from build123d import *

# Parameters (mm, degrees)
ESBO_O1_R                = 18
RESSALTO_EXTRUS_O1_DEPTH = 27
ESBO_O7_R                = 3.5
ESBO_O7_R_2              = 3
CORTE_EXTRUS_O3_DEPTH    = 5
ESBO_O13_R               = 3.5
ESBO_O13_R_2             = 1.25
CORTE_EXTRUS_O4_DEPTH    = 5
ESBO_O14_R               = 6.5
RESSALTO_EXTRUS_O2_DEPTH = 1.6
RESSALTO_EXTRUS_O4_DEPTH = 7
CORTE_EXTRUS_O5_DEPTH    = 7
ESBO_O21_R               = 1.25
RESSALTO_EXTRUS_O5_DEPTH = 7
CORTE_EXTRUS_O6_START    = -1
ESBO_O22_R               = 3.5
CORTE_EXTRUS_O6_DEPTH    = 1
ESBO_O23_R               = 2.5
RESSALTO_EXTRUS_O6_DEPTH = 17.5
FILETE2_R                = 0.5


with BuildPart() as part:
    # Esboço1 → Ressalto-extrusão1 (new, symmetric)
    with BuildSketch(Plane.XY):
        Circle(ESBO_O1_R)
    extrude(amount=RESSALTO_EXTRUS_O1_DEPTH, both=True)

    # Esboço7 → Corte-extrusão3 (cut)
    with BuildSketch(Plane(origin=(0, 0, -27), x_dir=(-1, 0, 0), z_dir=(0, 0, -1))):
        Circle(ESBO_O7_R)
        with Locations((0, 11.5)):
            Circle(ESBO_O7_R_2)
        with Locations((-8.131727984, 8.131727984)):
            Circle(ESBO_O7_R_2)
        with Locations((-11.5, 0)):
            Circle(ESBO_O7_R_2)
        with Locations((-8.131727984, -8.131727984)):
            Circle(ESBO_O7_R_2)
        with Locations((8.131727984, -8.131727984)):
            Circle(ESBO_O7_R_2)
        with Locations((11.5, 0)):
            Circle(ESBO_O7_R_2)
        with Locations((8.131727984, 8.131727984)):
            Circle(ESBO_O7_R_2)
    extrude(amount=-CORTE_EXTRUS_O3_DEPTH, mode=Mode.SUBTRACT)

    # Esboço13 → Corte-extrusão4 (cut)
    with BuildSketch(Plane.XY.offset(27)):
        with Locations((-11, 0)):
            Circle(ESBO_O13_R)
        with Locations((11, 0)):
            Circle(ESBO_O13_R)
        with Locations((0, 11)):
            Circle(ESBO_O13_R)
        with Locations((0, -11)):
            Circle(ESBO_O13_R)
        with Locations((-8.768124087, -8.768124087)):
            Circle(ESBO_O13_R_2)
        with Locations((6.363961031, -6.363961031)):
            Circle(ESBO_O13_R_2)
        with Locations((-6.363961031, 6.363961031)):
            Circle(ESBO_O13_R_2)
        with Locations((8.768124087, 8.768124087)):
            Circle(ESBO_O13_R_2)
    extrude(amount=-CORTE_EXTRUS_O4_DEPTH, mode=Mode.SUBTRACT)

    # Esboço14 → Ressalto-extrusão2 (add)
    with BuildSketch(Plane.XY.offset(27)):
        Circle(ESBO_O14_R)
    extrude(amount=RESSALTO_EXTRUS_O2_DEPTH)

    # Esboço17 → Ressalto-extrusão4 (add)
    with BuildSketch(Plane(origin=(0, 0, -27), x_dir=(-1, 0, 0), z_dir=(0, 0, -1))):
        with BuildLine():
            ThreePointArc((-3.463586585, -14.296345868), (0, -14.709926486), (3.463586585, -14.296345868))
            ThreePointArc((3.463586585, -14.296345868), (4.825973045, -12.062760604), (2.592387781, -10.700374144))
            ThreePointArc((2.592387781, -10.700374144), (0, -11.009926486), (-2.592387781, -10.700374144))
            ThreePointArc((-2.592387781, -10.700374144), (-4.825973045, -12.062760604), (-3.463586585, -14.296345868))
        make_face()
    extrude(amount=RESSALTO_EXTRUS_O4_DEPTH)

    # Esboço18 → Corte-extrusão5 (cut)
    with BuildSketch(Plane(origin=(0, 0, -34), x_dir=(-1, 0, 0), z_dir=(0, 0, -1))):
        with BuildLine():
            ThreePointArc((-3.392948844, -14.004780593), (0, -14.409926486), (3.392948844, -14.004780593))
            ThreePointArc((3.392948844, -14.004780593), (4.53440777, -12.133398345), (2.663025521, -10.991939419))
            ThreePointArc((2.663025521, -10.991939419), (0, -11.309926486), (-2.663025521, -10.991939419))
            ThreePointArc((-2.663025521, -10.991939419), (-4.53440777, -12.133398345), (-3.392948844, -14.004780593))
        make_face()
    extrude(amount=-CORTE_EXTRUS_O5_DEPTH, mode=Mode.SUBTRACT)

    # Esboço21 → Ressalto-extrusão5 (add)
    with BuildSketch(Plane(origin=(0, 0, -27), x_dir=(-1, 0, 0), z_dir=(0, 0, -1))):
        with Locations((-3.027987183, -12.498360006)):
            Circle(ESBO_O21_R)
        with Locations((3.027987183, -12.498360006)):
            Circle(ESBO_O21_R)
        with Locations((0, -12.859926486)):
            Circle(ESBO_O21_R)
    extrude(amount=RESSALTO_EXTRUS_O5_DEPTH)

    # Esboço22 → Corte-extrusão6 (cut)
    with BuildSketch(Plane.XY.offset(28.6).offset(CORTE_EXTRUS_O6_START)):
        with Locations(Location((0, 0, 0), (0, 0, 180))):
            Circle(ESBO_O22_R)
    extrude(amount=CORTE_EXTRUS_O6_DEPTH, mode=Mode.SUBTRACT)

    # Esboço23 → Ressalto-extrusão6 (add)
    with BuildSketch(Plane.XY.offset(27.6)):
        Circle(ESBO_O23_R)
    extrude(amount=RESSALTO_EXTRUS_O6_DEPTH)

    # Filete2
    filete2_edges = [part.edges().sort_by_distance(p)[0] for p in [
        (-2.5, 0, 45.1),
    ]]
    fillet(filete2_edges, radius=FILETE2_R)


solid = part.part
Can you work these out from the model? Positions are in its coordinate system, mm. A direction names the side the tool comes from. Coordinates: 2 decimals unless noted, no trailing zeros. Loops run counter-clockwise (first coordinate to the right, second up) from the corner with the lowest first, then second, coordinate; pieces in that order, holes last. Notation, with made-up numbers: (-35, 41) - (-15, 41) arc R16 ccw to (-15, 70) - close; hole circle Ø7 at (-37.75, 35). An arc over 180 degrees is marked (long way). Answer as a JSON object with one key per item and string values. Group by question number.
Item 1: If we section it at A-A (z = -18): List the corners of the cut face in (x, y) for me, plus the area to 3 significant figures.
Item 2: If we mould it in two halves opening along X, with no side actions, what happens to faces 4 (the face through (3, -12, -34)), 5 (the face through (9.923, 8.289, 24.535)), 6 (the face through (-5.158, -3.955, 27.789))? For each: released by +X, released by -X, zero draft, split by the parting line, or undercut.
Item 3: If I drill on L1, parallel to Y at x = 0, z = 24; L2, parallel to Z at x = 5, y = 16; L3, parallel to Z at x = 0, y = 0, over which ranges is the centre line in solid material (lowest first)? Write a range as from..to.
Item 4: On a 3-axis mill with a long thin cutter (end or side, diameter ignored), from which of +Z, -Z, +X, -X, +Y, -Y can I reach the whole of each face in a straight line? I mean faces 1 (the face through (0, 0, 45.1)), 2 (the face through (6, -6, 22)), 3 (the face through (0.16, -11.62, -30.45)). Say none if no direction works.
Item 5: For pin 1 (1.5 mm diameter, centred on x = -6.5, y = -13.5, fed in from -Z); pin 2 (12 mm diameter, centred on x = -1.5, z = -25.5, fed in from +Y); pin 3 (4 mm diameter, centred on x = -13, z = -13, fed in from +Y), each with a flat end and sliding along its axis, tell me the tip position at first contact or that it passes through.
Item 6: If we section it at B-B (z = 38.5): List the corners of the cut face in (x, y) for me, plus the area to 3 significant figures.
Returned:
{
 "1": {"outline": "circle Ø36 at (0, 0)", "area": "1,020 mm²"},
 "2": {"face 4": "zero draft", "face 5": "undercut", "face 6": "split by the parting line"},
 "3": {"L1": "y = -18..-14.5, -7.5..7.5, 14.5..18", "L2": "z = -27..27", "L3": "z = -22..45.1"},
 "4": {"face 1": "+Z, +X, -X, +Y, -Y", "face 2": "+Z", "face 3": "-Z"},
 "5": {"pin 1": "stops at z = -27", "pin 2": "stops at y = 18", "pin 3": "stops at y = 14.25"},
 "6": {"outline": "circle Ø5 at (0, 0)", "area": "19.6 mm²"}
}
